Could you check a few things on this model? Use its own coordinates, in mm. A direction names the side the tool comes from. Give positions to 0.01 mm unless a question says otherwise; leave off trailing zeros. Order: outer loops, then holes, each group sorted by start corner. A loop starts at its lowest first (then second) coordinate and runs counter-clockwise, first axis right, second up. Notation, with made-up numbers: (47.5, -21.75) - (69.5, -21.75) arc R17 cw to (69.5, 3.25) - close; hole circle Ø3 at (-17.75, 70). An arc over 180 degrees is marked (long way). Put each result on its own line as item: value.
from build123d import *
from OCP.BRepFilletAPI import BRepFilletAPI_MakeChamfer

# Parameters (mm, degrees)
SKIZZE1_W                                 = 10.16
SKIZZE1_H                                 = 8.765
SKIZZE1_H_2                               = 6.335
SKIZZE1_R                                 = 1.875
AUFSATZ_LINEAR_AUSTRAGEN1_DEPTH           = 4.195
SCHNITT_LINEAR_AUSTRAGEN1_DEPTH           = 14.821249039
SCHNITT_LINEAR_AUSTRAGEN1_DEPTH_BACK      = 14.821249039
SCHNITT_LINEAR_AUSTRAGEN2_DEPTH           = 14.821249039
SCHNITT_LINEAR_AUSTRAGEN2_DEPTH_BACK      = 14.821249039
AUFSATZ_LINEAR_AUSTRAGEN2_DEPTH           = 0.47
SKIZZE6_R                                 = 0.9
SCHNITT_LINEAR_AUSTRAGEN3_DEPTH           = 27.52093984
SCHNITT_LINEAR_AUSTRAGEN3_DRAFT           = -4
SCHNITT_LINEAR_AUSTRAGEN3_PROFILE_2_DEPTH = 27.52093984
SCHNITT_LINEAR_AUSTRAGEN3_PROFILE_2_DRAFT = -4
FASE1_SIZE                                = 2
FASE1_SIZE2                               = 1.154700538


with BuildPart() as part:
    # Skizze1 → Aufsatz-Linear austragen1 (new body)
    # profile 1 of 2: a face of its own
    with BuildSketch(Plane.XY):
        with Locations((0, -7.7675)):
            Rectangle(SKIZZE1_W, SKIZZE1_H)
    # profile 2 of 2: a face of its own
    with BuildSketch(Plane.XY):
        with Locations((0, -0.2175)):
            Rectangle(SKIZZE1_W, SKIZZE1_H_2)
        Circle(SKIZZE1_R, mode=Mode.SUBTRACT)
    extrude(amount=AUFSATZ_LINEAR_AUSTRAGEN1_DEPTH)

    # Skizze3 → Schnitt-Linear austragen1 (cut, two sides: drawn at the far end of the back side and taken through both)
    with BuildSketch(Plane(origin=(0, 0, 0), x_dir=(0, 0, -1), z_dir=(1, 0, 0)).offset(-SCHNITT_LINEAR_AUSTRAGEN1_DEPTH_BACK)):
        Polygon((-1.27, 43.960404594), (-1.27, 2.95), (-1.27, -3.385), (-4.195, -3.640904341), (-4.195, -12.029725883), (-2.475, -12.15), (0, -11.97693114), (40.91050531, -9.116189929), (-23.302349016, -60.146793289), (-65.482854325, -7.070198766), align=None)
    extrude(amount=SCHNITT_LINEAR_AUSTRAGEN1_DEPTH + SCHNITT_LINEAR_AUSTRAGEN1_DEPTH_BACK, mode=Mode.SUBTRACT)

    # Skizze4 → Schnitt-Linear austragen2 (cut, two sides: drawn at the far end of the back side and taken through both)
    with BuildSketch(Plane(origin=(0, 0, 0), x_dir=(1, 0, 0), z_dir=(0, 1, 0)).offset(-SCHNITT_LINEAR_AUSTRAGEN2_DEPTH_BACK)):
        Polygon((-7.252588261, 29.799459635), (-5.08, -1.27), (-4.875464075, -4.195), (4.875464075, -4.195), (5.08, -1.27), (7.252588261, 29.799459635), (7.252588261, -32.491196543), (-7.252588261, -32.491196543), align=None)
    extrude(amount=SCHNITT_LINEAR_AUSTRAGEN2_DEPTH + SCHNITT_LINEAR_AUSTRAGEN2_DEPTH_BACK, mode=Mode.SUBTRACT)

    # Skizze5 → Aufsatz-Linear austragen2 (add)
    with BuildSketch(Plane.XY.offset(2.475)):
        Polygon((-3.63, -11.15), (-3.63, -18.5), (-3.25, -18.5), (-3.25, -25.605192379), (-3.1, -25.865), (-2.7, -25.865), (-2.55, -25.605192379), (-2.55, -18.5), (-2.17, -18.5), (-2.17, -11.15), align=None)
        Polygon((-0.73, -11.15), (-0.73, -18.5), (-0.35, -18.5), (-0.35, -25.605192379), (-0.2, -25.865), (0.2, -25.865), (0.35, -25.605192379), (0.35, -18.5), (0.73, -18.5), (0.73, -11.15), align=None)
        Polygon((2.17, -11.15), (2.17, -18.5), (2.55, -18.5), (2.55, -25.605192379), (2.7, -25.865), (3.1, -25.865), (3.25, -25.605192379), (3.25, -18.5), (3.63, -18.5), (3.63, -11.15), align=None)
    extrude(amount=AUFSATZ_LINEAR_AUSTRAGEN2_DEPTH)


with BuildPart() as schnitt_linear_austragen3_tool:
    # Skizze6 → Schnitt-Linear austragen3 (with draft: the straight prism first)
    with BuildSketch(Plane.XY.offset(1.27)):
        with Locations((-5.08, -9.385)):
            Circle(SKIZZE6_R)
    extrude(amount=SCHNITT_LINEAR_AUSTRAGEN3_DEPTH)
    # Schnitt-Linear austragen3: the draft: its side faces are tilted about the plane it starts from
    schnitt_linear_austragen3_sides = [schnitt_linear_austragen3_tool.faces().sort_by_distance(p)[0] for p in [
        (-5.98, -9.385, 15.03046992),
    ]]
    draft(schnitt_linear_austragen3_sides, Plane.XY.offset(1.27), SCHNITT_LINEAR_AUSTRAGEN3_DRAFT)


with BuildPart() as part_1:
    add(part.part)

    # Schnitt-Linear austragen3: cut by schnitt_linear_austragen3_tool
    add(schnitt_linear_austragen3_tool.part, mode=Mode.SUBTRACT)


with BuildPart() as schnitt_linear_austragen3_profile_2_tool:
    # Skizze6 → Schnitt-Linear austragen3 profile 2 (with draft: the straight prism first)
    with BuildSketch(Plane.XY.offset(1.27)):
        with Locations((5.08, -9.385)):
            Circle(SKIZZE6_R)
    extrude(amount=SCHNITT_LINEAR_AUSTRAGEN3_PROFILE_2_DEPTH)
    # Schnitt-Linear austragen3 profile 2: the draft: its side faces are tilted about the plane it starts from
    schnitt_linear_austragen3_profile_2_sides = [schnitt_linear_austragen3_profile_2_tool.faces().sort_by_distance(p)[0] for p in [
        (4.18, -9.385, 15.03046992),
    ]]
    draft(schnitt_linear_austragen3_profile_2_sides, Plane.XY.offset(1.27), SCHNITT_LINEAR_AUSTRAGEN3_PROFILE_2_DRAFT)


with BuildPart() as part_2:
    add(part_1.part)

    # Schnitt-Linear austragen3 profile 2: cut by schnitt_linear_austragen3_profile_2_tool
    add(schnitt_linear_austragen3_profile_2_tool.part, mode=Mode.SUBTRACT)

    # Fase1: one chamfer whose edges measure the first distance from different faces: ONE call of the kernel's chamfer builder (chamfer() names one face for all edges)
    fase1_edges_1 = [part_2.edges().sort_by_distance(p)[0] for p in [
        (-5.08, 2.95, 0.635),
    ]]
    fase1_side_1 = [part_2.faces().sort_by_distance(p)[0] for p in [
        (-5.08, -4.535689282, 0.635627783),
    ]]
    fase1_edges_2 = [part_2.edges().sort_by_distance(p)[0] for p in [
        (5.08, 2.95, 0.635),
    ]]
    fase1_side_2 = [part_2.faces().sort_by_distance(p)[0] for p in [
        (5.08, -4.535689282, 0.635627783),
    ]]
    fase1 = BRepFilletAPI_MakeChamfer(part_2.part.solid().wrapped)
    for e in fase1_edges_1:
        fase1.Add(FASE1_SIZE, FASE1_SIZE2, e.wrapped, fase1_side_1[0].wrapped)  # the first distance lies on this face
    for e in fase1_edges_2:
        fase1.Add(FASE1_SIZE, FASE1_SIZE2, e.wrapped, fase1_side_2[0].wrapped)  # the first distance lies on this face
    add(Compound.cast(fase1.Shape()), mode=Mode.REPLACE)


solid = part_2.part
1) I'm going to push flat-ended pins straight in: pin 1 (0.7 mm diameter, centred on x = -5, y = -9, fed in from +Z); pin 2 (0.7 mm diameter, centred on x = -0.5, y = -18.5, fed in from +Z) (3 decimals); pin 3 (2 mm diameter, centred on x = 0, y = 0, fed in from +Z); pin 4 (0.5 mm diameter, centred on y = -16.5, z = 2.5, fed in from +X). Where does each tip first touch, or does it pass through?
Filled in:
pin 1: stops at z = 1.27
pin 2: stops at z = 2.945
pin 3: passes through
pin 4: stops at x = 3.63
2) We'd pull the mould along Y, two halves only. Please class faces 1 (the flat face through (4.7, -9.4, 1.27)), 2 (the flat face through (-4.98, -5.97, 2.71)), 3 (the flat face through (-0.07, -3.51, 2.71)): pulls with the +Y half, pulls with the -Y half, needs draft (parallel to the pull), parting line crosses it, or undercut.
Filled in:
face 1: undercut
face 2: needs draft
face 3: pulls with the +Y half
3) Which directions (+Z, -Z, +X, -X, +Y, -Y) give clear straight access to the entire face, cutting with the end or side of a thin tool? Please do faces 4 (the flat face through (3, -17, 2.475)), 5 (the flat face through (3, -17, 2.945)), 6 (the flat face through (4.976, -11.231, 2.753)), 7 (the flat face through (-4.7, -9.4, 1.27)).
Filled in:
face 4: -Z, +X, -X, -Y
face 5: +Z, +X, -X, -Y
face 6: +Z, +X, +Y, -Y
face 7: +Z, -X
4) Suppose I cut it at B-B, the plane y = -17.5. List the corners of the cut face in (x, z) for me (3 decimals), and give its area (3 significant figures).
Filled in:
outline: (-3.63, 2.475) - (-2.17, 2.475) - (-2.17, 2.945) - (-3.63, 2.945) - close; (-0.73, 2.475) - (0.73, 2.475) - (0.73, 2.945) - (-0.73, 2.945) - close; (2.17, 2.475) - (3.63, 2.475) - (3.63, 2.945) - (2.17, 2.945) - close
area: 2.06 mm^2
5) Suppose I cut it at A-A, the plane y = 0. List the corners of the cut face in (x, z) for me (3 decimals).
Filled in:
outline: (-5.08, 0) - (-1.875, 0) - (-1.875, 1.27) - (-5.08, 1.27) - close; (1.875, 0) - (5.08, 0) - (5.08, 1.27) - (1.875, 1.27) - close
6) If I drill on line 1 (Y direction, x = 0, z = 0.7) (3 decimals); line 2 (X direction, y = 0, z = 0.55) (3 decimals); line 3 (Z direction, x = 4.25, y = -9.5), over which ranges is the centre line in solid material (lowest first)? Write a range as [from, to].
Filled in:
line 1: y = [-12.026, -1.875], [1.875, 2.95]
line 2: x = [-5.08, -1.875], [1.875, 5.08]
line 3: z = [0, 1.27]
7) Suppose I cut it at C-C, the plane z = 1.55. List the corners of the cut face in (x, y) for me (1 decimal), and give its area (3 significant figures).
Filled in:
outline: (-5.1, -12.1) - (5.1, -12.1) - (5.1, -10.3) arc R0.9 cw to (5.1, -8.5) - (5.1, -3.4) - (-5.1, -3.4) - (-5.1, -8.5) arc R0.9 cw to (-5.1, -10.3) - close
area: 85.2 mm^2
